Geometry: final body of the model. Coordinates: model frame, mm. Face numbers are marked on the shaded views. Give positions to 0.01 mm unless a question says otherwise; leave off trailing zeros. Write each loop counter-clockwise with the first axis right and the second up, starting at its lowest first coordinate (ties: lowest second). Pieces come first, ordered by that corner, then holes. Notation, with made-up numbers: (70.25, -29) -> (109.25, -29) arc R3 cw to (109.25, -24) -> close; hole circle Ø4 at (-31.5, 65). An arc over 180 degrees is marked (long way). Answer in a Markdown table with one row per item. Add a question column.
Item 1: Section query B-B on y = 93.85. Output: boundary loops of the cut face in (x, z), plus the area to 3 significant figures.
Item 2: Draft query along Z for the marked faces 1, 2 and 3. Return one class per face: +Z half, -Z half, draft (parallel to the pull), parting line (faces both ways), or undercut.
Item 3: Section query C-C on x = 7.25. Output: boundary loops of the cut face in (y, z).
Item 4: Material intervals for probe 1 along Z at (x, y) = (2, 93.85); probe 2 along Y at (x, z) = (5.5, -24); probe 3 along Y at (x, z) = (0.75, -17), sorted ascending. Write a range as from..to.
Item 5: Section query A-A on z = -24.75. Output: boundary loops of the cut face in (x, y).
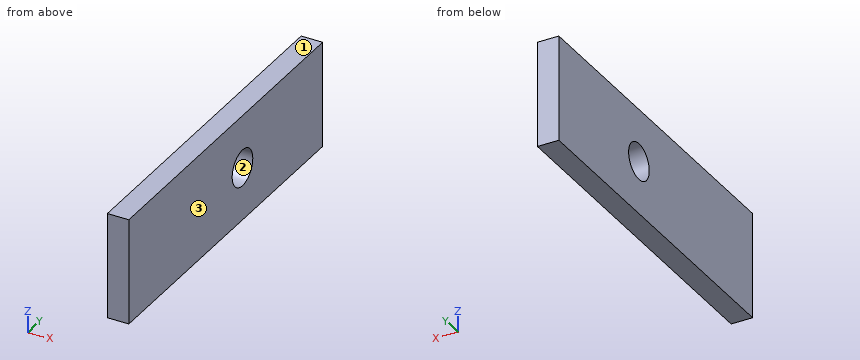
Autodesk Inventor part; units mm, degrees
ref_plane "YZ Plane" through (0, 0, 0) normal (1, 0, 0) x (0, 1, 0)
ref_plane "XZ Plane" through (0, 0, 0) normal (0, 1, 0) x (-1, 0, 0)
ref_plane "XY Plane" through (0, 0, 0) normal (0, 0, 1) x (1, 0, 0)
sketch "Sketch1" plane through (0, 0, 0) normal (1, 0, 0) x (0, 1, 0)
  line L0 (0, 0) -> (160, 0)
  line L1 (160, 0) -> (160, -49.5)
  line L2 (160, -49.5) -> (0, -49.5)
  line L3 (0, -49.5) -> (0, 0)
  line L4 (0, -24.75) -> (93.85, -24.75)
  circle A0 centre (93.85, -24.75) radius 8.5
  dimension "d0" = 160
  dimension "d1" = 49.5
  dimension "d2" = 93.85
  dimension "d3" = 17
extrude "Extrusion1" add sketch "Sketch1" along normal blind 10
properties part number "tallwall3"
Findings below:
| question | item | result |
|---|---|---|
| 1 | outline | (0, -49.5) -> (10, -49.5) -> (10, -33.25) -> (0, -33.25) -> close; (0, -16.25) -> (10, -16.25) -> (10, 0) -> (0, 0) -> close |
| 1 | area | 325 mm^2 |
| 2 | face 1 | +Z half |
| 2 | face 2 | undercut |
| 2 | face 3 | draft |
| 3 | outline | (0, -49.5) -> (160, -49.5) -> (160, 0) -> (0, 0) -> close; hole circle Ø17 at (93.85, -24.75) |
| 4 | probe 1 | z = -49.5..-33.25, -16.25..0 |
| 4 | probe 2 | y = 0..85.38, 102.32..160 |
| 4 | probe 3 | y = 0..90.36, 97.34..160 |
| 5 | outline | (0, 0) -> (10, 0) -> (10, 85.35) -> (0, 85.35) -> close; (0, 102.35) -> (10, 102.35) -> (10, 160) -> (0, 160) -> close |
